```python
from build123d import *

# Parameters (mm, degrees)
SKETCH1_R          = 2.375
EXTRUDE1_DEPTH     = 1.2
FILLET1_R          = 1
CUT_EXTRUDE1_DEPTH = 0.7
CUT_EXTRUDE1_DRAFT = -25
SKETCH3_R          = 1.1
EXTRUDE2_DEPTH     = 4.7625


with BuildPart() as part:
    # Sketch1 → Extrude1 (new body)
    with BuildSketch(Plane.XY):
        Circle(SKETCH1_R)
    extrude(amount=EXTRUDE1_DEPTH)

    # Fillet1
    fillet1_edges = [part.edges().sort_by_distance(p)[0] for p in [
        (-2.375, 0, 1.2),
    ]]
    fillet(fillet1_edges, radius=FILLET1_R)


with BuildPart() as cut_extrude1_tool:
    # Sketch2 → Cut-Extrude1 (with draft: the straight prism first)
    with BuildSketch(Plane.XY.offset(1.2)):
        Polygon((-0.4, 0.4), (-1.2, 0.4), (-1.2, -0.4), (-0.4, -0.4), (-0.4, -1.2), (0.4, -1.2), (0.4, -0.4), (1.2, -0.4), (1.2, 0.4), (0.4, 0.4), (0.4, 1.2), (-0.4, 1.2), align=None)
    extrude(amount=-CUT_EXTRUDE1_DEPTH)
    # Cut-Extrude1: the draft: its side faces are tilted about the plane it starts from
    cut_extrude1_sides = [cut_extrude1_tool.faces().sort_by_distance(p)[0] for p in [
        (-0.8, 0.4, 0.85),
        (-1.2, 0, 0.85),
        (-0.8, -0.4, 0.85),
        (-0.4, -0.8, 0.85),
        (0, -1.2, 0.85),
        (0.4, -0.8, 0.85),
        (0.8, -0.4, 0.85),
        (1.2, 0, 0.85),
        (0.8, 0.4, 0.85),
        (0.4, 0.8, 0.85),
        (0, 1.2, 0.85),
        (-0.4, 0.8, 0.85),
    ]]
    draft(cut_extrude1_sides, Plane.XY.offset(1.2), CUT_EXTRUDE1_DRAFT)


with BuildPart() as part_1:
    add(part.part)

    # Cut-Extrude1: cut by cut_extrude1_tool
    add(cut_extrude1_tool.part, mode=Mode.SUBTRACT)

    # Sketch3 → Extrude2 (add)
    with BuildSketch(Plane(origin=(0, 0, 0), x_dir=(-1, 0, 0), z_dir=(0, 0, -1))):
        with Locations(Location((0, 0, 0), (0, 0, 180))):
            Circle(SKETCH3_R)
    extrude(amount=EXTRUDE2_DEPTH)


solid = part_1.part
```
Model file for the job. Use its own axes, mm. A direction names the side the tool comes from. Give positions to 0.01 mm unless a question says otherwise; leave off trailing zeros. Loops run counter-clockwise (first coordinate to the right, second up) from the corner with the lowest first, then second, coordinate; pieces in that order, holes last. Notation, with made-up numbers: (57.5, -20) -> (83.5, -20) arc R12 cw to (83.5, -11) -> close; hole circle Ø11 at (30, 12). An arc over 180 degrees is marked (long way). Use CSV: the item, a comma, the result in double quotes. Start each with the question number.
1) Tool access for faces 1 (the flat face through (1, 1, 0)), 2 (the flat face through (0, 0, -4.762)): list every direction of +Z, -Z, +X, -X, +Y, -Y with a clear straight run to the whole face (end or side of a thin tool).
2) Wall check: line 1 (Z direction, x = -0.85, y = 0.85); line 2 (Y direction, x = -0.2, z = -0.8); line 3 (X direction, y = 1.7, z = 0.85). Give the ranges that are in metal, low to high.
3) Slice it at C-C on z = -4.1. Give the cut face in (x, y), plus the area to 3 significant figures.
4) Flat gauge pins, fed straight in: pin 1 Ø1.9 at (x, y) = (0.5, 0) entering from +Z; pin 2 Ø1.5 at (x, z) = (-1, -3) entering from -Y. Where does each tip first touch, or does it go through?
Computed values:
1,face 1,"-Z"
1,face 2,"-Z, +X, -X, +Y, -Y"
2,line 1,"z = 0 to 1.2"
2,line 2,"y = -1.08 to 1.08"
2,line 3,"x = -1.29 to 1.29"
3,outline,"circle Ø2.2 at (0, 0)"
3,area,"3.80 mm^2"
4,pin 1,"stops at z = 1.2"
4,pin 2,"stops at y = -1.07"
